Autodesk Inventor part; units mm, degrees
ref_plane "YZ Plane" through (0, 0, 0) normal (1, 0, 0) x (0, 1, 0)
ref_plane "XZ Plane" through (0, 0, 0) normal (0, 1, 0) x (-1, 0, 0)
ref_plane "XY Plane" through (0, 0, 0) normal (0, 0, 1) x (1, 0, 0)
sketch "Sketch1" plane through (0, 0, 0) normal (0, 1, 0) x (-1, 0, 0)
  line L0 (25, 10) -> (-25, 10)
  line L1 (-25, 10) -> (-25, -10)
  line L2 (-25, -10) -> (25, -10)
  line L3 (25, -10) -> (25, 10)
  line L4 (25, 10) -> (-25, -10) construction
  line L5 (-25, 10) -> (25, -10) construction
  point P0 (0, 0)
  dimension "d0" = 50
  dimension "d1" = 20
extrude "Extrusion1" add sketch "Sketch1" along normal blind 5
sketch "Sketch2" plane through (0, 0, 0) normal (0, -1, 0) x (1, 0, 0)
  line L0 (-25, -10) -> (-25, 10)
  line L1 (-25, 10) -> (-20, 10)
  line L2 (-25, 10) -> (25, 10)
  line L3 (-20, 10) -> (-20, -10)
  line L4 (25, -10) -> (-25, -10)
  line L5 (-25, -10) -> (-20, -10)
  line L6 (-25, 10) -> (-25, -10)
  point P0 (0, 0)
  dimension "d4" = 5
extrude "Extrusion2" add sketch "Sketch2" along normal blind 30
sketch "Sketch3" plane through (-20, 0, 10) normal (1, 0, 0) x (0, 0, -1)
  point P0 (10, 0)
sketch "Sketch4" plane through (-25, 5, 10) normal (0, 0, 1) x (1, 0, 0)
  line L0 (5, -5) -> (50, -5)
  line L1 (50, -5) -> (50, 0)
  line L2 (0, 0) -> (50, 0)
  line L3 (0, -35) -> (0, 0)
  line L4 (5, -35) -> (0, -35)
  line L5 (5, -5) -> (5, -35)
  line L6 (25, -5) -> (5, -17.5)
  dimension "d7" = 10.6
extrude "Extrusion3" add sketch "Sketch4" against normal blind 5 contours L0 L6 L5
mirror "Mirror1" about plane through (0, 0, 0) normal (0, 0, 1) of "Extrusion3"
sketch "Sketch5" plane through (-20, -30, 10) normal (1, 0, 0) x (0, 0, -1)
  circle A0 centre (10, 17.5) radius 4
  line L0 (0, 30) -> (20, 30)
  line L1 (0, 17.5) -> (0, 0)
  point P0 (10, 30)
  point P1 (10, 30)
  dimension "d10" = 8
  dimension "d11" = 12.5
  dimension "d12" = 10
extrude "Extrusion4" cut sketch "Sketch5" against normal blind 5
fillet "Fillet1" radius 2 2 edges at (-10, -6.25, 5) (-10, -6.25, -5)
fillet "Fillet2" radius 2 8 edges at (12.5, 0, -10) (-10, -6.25, -10) (25, 0, 0) (12.5, 0, 10) (-10, -6.25, 10) (-20, -21.25, -10) (-20, -30, 0) (-20, -21.25, 10)
Work out the finished part from the listing and answer in its coordinate system (mm). A direction names the side the tool comes from. Give positions to 0.01 mm unless a question says otherwise; leave off trailing zeros. Write each loop counter-clockwise with the first axis right and the second up, starting at its lowest first coordinate (ties: lowest second). Pieces come first, ordered by that corner, then holes.
Q1. The part is cut by section D-D on y = -19.5. Give the vertices of the cut face in (x, z), and give its area (3 significant figures).
Answer:
outline: (-25, -10) - (-22, -10) arc R2 ccw to (-20, -8) - (-20, 8) arc R2 ccw to (-22, 10) - (-25, 10) - close
area: 98.3 mm2
Q2. The part is cut by section A-A on z = 0. Give the vertices of the cut face in (x, y).
Answer:
outline: (-25, -30) - (-22, -30) arc R2 ccw to (-20, -28) - (-20, -16.5) - (-25, -16.5) - close; (-25, -8.5) - (-20, -8.5) - (-20, 0) - (23, 0) arc R2 ccw to (25, 2) - (25, 5) - (-25, 5) - close
Q3. Given pin 1 (3 mm diameter, centred on y = -8.5, z = 5.5, fed in from +X); pin 2 (1.5 mm diameter, centred on x = 17, y = -2, fed in from +Z); pin 3 (10 mm diameter, centred on x = -5, z = 2.5, fed in from -Y); pin 4 (8 mm diameter, centred on x = 14.5, z = 3.5, fed in from -Y), each flat-ended and moving along its own axis, determine where each tip first touches the part or whether it passes through.
Answer:
pin 1: stops at x = -11.79
pin 2: passes through
pin 3: stops at y = -5.04
pin 4: stops at y = 0
Q4. A tool of negligible diameter and unlimited length cuts with its end or side. For faces 4 (the face through (-20.57, -20.83, 9.4)), 5 (the face through (7, 0, 0)), 6 (the face through (-20.6, -20.83, -9.43)), 7 (the face through (-13, -3, 10)), 8 (the face through (-9.86, -6.163, 7.507)), from which of +Z, -Z, +X, -X, +Y, -Y can it reach the whole face along a straight path? Write none if from no direction.
Answer:
face 4: +Z, +X, -Y
face 5: +X, -Y
face 6: -Z, +X, -Y
face 7: +Z, +X, -X, +Y, -Y
face 8: +Z, -Z, +X, -Y
Q5. The part is cut by section C-C on x = 14. Give the vertices of the cut face in (y, z), and give its area (3 significant figures).
Answer:
outline: (0, -8) arc R2 ccw to (2, -10) - (5, -10) - (5, 10) - (2, 10) arc R2 ccw to (0, 8) - close
area: 98.3 mm2
Q6. Straight lines are drawn through the part: L1, parallel to Y at x = -22.4, z = 0; L2, parallel to Z at x = -18.5, y = -9; L3, parallel to Y at x = -1, z = -4.75. For each, find the intervals that lie inside material, in ascending order.
Answer:
L1: y = -30 to -16.5, -8.5 to 5
L2: z = -10 to -5, 5 to 10
L3: y = 0 to 5
Q7. For a pull along Z with two mould halves and no side action, classify faces 1 (the face through (12.03, 0.6, -9.43)), 2 (the face through (-10.44, -5.85, -5.6)), 3 (the face through (25, 3, 0)) as released by +Z, released by -Z, zero draft, split by the parting line, or undercut.
Answer:
face 1: released by -Z
face 2: undercut
face 3: zero draft
Q8. The part is cut by section B-B on y = -14.5. Give the vertices of the cut face in (x, z), and give its area (3 significant figures).
Answer:
outline: (-25, -10) - (-22, -10) arc R2 ccw to (-20, -8) - (-20, -3.46) - (-25, -3.46) - close; (-25, 3.46) - (-20, 3.46) - (-20, 8) arc R2 ccw to (-22, 10) - (-25, 10) - close
area: 63.6 mm2
